Autodesk Inventor part; units mm, degrees
ref_plane "YZ Plane" through (0, 0, 0) normal (1, 0, 0) x (0, 1, 0)
ref_plane "XZ Plane" through (0, 0, 0) normal (0, 1, 0) x (-1, 0, 0)
ref_plane "XY Plane" through (0, 0, 0) normal (0, 0, 1) x (1, 0, 0)
sketch "スケッチ1" plane through (0, 0, 0) normal (0, 0, 1) x (1, 0, 0)
  circle A0 centre (2.8, 0) radius 2.8
  line L0 (2.8, 0) -> (0, 0)
  circle A1 centre (0, 2.8) radius 2.8
  circle A2 centre (-2.8, 0) radius 2.8
  circle A3 centre (0, -2.8) radius 2.8
  circle A4 centre (2.8, 0) radius 1.5
  circle A5 centre (0, 2.8) radius 1.5
  circle A6 centre (-2.8, 0) radius 1.5
  circle A7 centre (0, -2.8) radius 1.5
  circle A8 centre (0, 0) radius 5
  circle A9 centre (0, 5) radius 1.5
  circle A10 centre (-5, 0) radius 1.5
  circle A11 centre (0, -5) radius 1.5
  circle A12 centre (5, 0) radius 1.5
  point P0 (-1.483, -4.775)
  point P1 (1.483, -4.775)
  point P2 (-4.775, -1.483)
  point P3 (-4.775, 1.483)
  point P4 (4.775, 1.483)
  point P5 (4.775, -1.483)
  point P6 (-1.483, 4.775)
  point P7 (1.483, 4.775)
  dimension "d12" = 10
  dimension "d1" = 5.6
  dimension "d4" = 360
  dimension "d7" = 3
  dimension "d10" = 360
  dimension "d15" = 3
  dimension "d18" = 360
extrude "押し出し1" add sketch "スケッチ1" along normal blind 4 contours A8 A12 A4 A1 A0 | A0 A1 A8 | A8 A12 A4 | A8 A3 A0 | A0 A3 A4 A12 A8 | A1 A4 A0 A5 | A0 A5 A9 A8 A1 | A3 A8 A11 A7 A0 | A0 A7 A3 A4 | A9 A5 A8 | A8 A11 A7 | A0 A2 A5 | A4 L0 A1 | A9 A5 A2 A1 A8 | A7 A2 A0 | A3 L0 A4 | A8 A3 A2 A7 A11 | A3 A6 A1 | A1 A6 A2 A5 | A2 A7 A3 A6 | A1 A2 A8 | A8 A2 A3 | A1 A6 A10 A8 A2 | A2 A8 A10 A6 A3 | A10 A6 A8
properties part number "カムL4" material "アセタール樹脂、白"
Geometry check sheet. Reference: the model listing, model coordinates, mm. Give positions to 0.01 mm unless a question says otherwise; leave off trailing zeros. Loops run counter-clockwise (first coordinate to the right, second up) from the corner with the lowest first, then second, coordinate; pieces in that order, holes last. Notation, with made-up numbers: M -35,82.5 L -22,82.5 A19 cw -22,104.5 Z; hole C 6.25,-11 d5. An arc over 180 degrees is marked long. Write item = value, one per line.
(1) Release check for a two-part mould opening along X. For faces 1 (the face through (0, 0, 0)), 2 (the face through (-1.08, 4.88, 1.97)), 3 (the face through (1.3, -0.07, 1.97)) record: released by +X, released by -X, zero draft, split by the parting line, or undercut.
Answer below:
face_1 = zero draft
face_2 = split by the parting line
face_3 = undercut
(2) Gauge pin test, flat ends, axial feed: pin 1 Ø2.5 at (x, y) = (2.8, 0) entering from -Z; pin 2 Ø6 at (x, y) = (-2, -1.5) entering from -Z; pin 3 Ø2 at (y, z) = (4, 3) entering from +X. Record the tip position at first contact, or that the pin passes through.
Answer below:
pin_1 = through
pin_2 = 0
pin_3 = 4
(3) Sectioned sample at D-D, the plane z = 3.3. Record the cut outline in (x, y).
Answer below:
outline = C 0,0 d10; hole C -2.8,0 d3; hole C 0,-2.8 d3; hole C 0,2.8 d3; hole C 2.8,0 d3
(4) Sectioned sample at A-A, the plane y = 3. Record the cut outline in (x, z), plus the area to 3 significant figures.
Answer below:
outline = M -4,0 L -1.49,0 L -1.49,4 L -4,4 Z; M 1.49,0 L 4,0 L 4,4 L 1.49,4 Z
area = 20.1 mm2
(5) Sectioned sample at B-B, the plane x = 0. Record the cut outline in (y, z), plus the area to 3 significant figures.
Answer below:
outline = M -5,0 L -4.3,0 L -4.3,4 L -5,4 Z; M -1.3,0 L 1.3,0 L 1.3,4 L -1.3,4 Z; M 4.3,0 L 5,0 L 5,4 L 4.3,4 Z
area = 16.0 mm2
(6) Material ranges on line 1 (X direction, y = 0, z = 1.3); line 2 (Y direction, x = 0.5, z = 3.1), recorded low to high. Write a range as [from, to].
Answer below:
line_1 = [-5, -4.3], [-1.3, 1.3], [4.3, 5]
line_2 = [-4.97, -4.21], [-1.39, 1.39], [4.21, 4.97]
(7) Sectioned sample at C-C, the plane x = 2.8. Record the cut outline in (y, z).
Answer below:
outline = M -4.14,0 L -1.5,0 L -1.5,4 L -4.14,4 Z; M 1.5,0 L 4.14,0 L 4.14,4 L 1.5,4 Z
